from build123d import *

# Parameters (mm, degrees)
BOSS_EXTRU_1_DEPTH      = 22
D_GAGEMENT_M21_D        = 2.4
ESQUISSE5_W             = 22
ESQUISSE5_H             = 10
BOSS_EXTRU_2_DEPTH      = 5
CONG_1_R                = 10
CONG_3_R                = 1
ENL_V_MAT_EXTRU_2_DEPTH = 3
ESQUISSE12_R            = 1.9376057
ENL_V_MAT_EXTRU_3_DEPTH = 37.235341952
ESQUISSE13_R            = 2.5
ENL_V_MAT_EXTRU_4_DEPTH = 2
ESQUISSE15_R            = 2.5
ENL_V_MAT_EXTRU_5_DEPTH = 7


with BuildPart() as part:
    # Esquisse1 → Boss.-Extru.1 (new body)
    with BuildSketch(Plane.XY):
        with BuildLine():
            Line((0, 10), (0, 0))
            Line((0, 0), (6, 0))
            ThreePointArc((6, 0), (11, 5), (16, 0))
            Line((16, 0), (22, 0))
            Line((22, 0), (22, 10))
            Line((22, 10), (0, 10))
        make_face()
    extrude(amount=BOSS_EXTRU_1_DEPTH)

    # Dégagement M21 (through all)
    with Locations(Plane(origin=(0, 10, 0), x_dir=(1, 0, 0), z_dir=(0, 1, 0))):
        with Locations((11, -6), (11, -18), (3, -12), (19, -12)):
            Hole(D_GAGEMENT_M21_D / 2)

    # Esquisse5 → Boss.-Extru.2 (add)
    with BuildSketch(Plane.XY.offset(22)):
        with Locations((11, 5)):
            Rectangle(ESQUISSE5_W, ESQUISSE5_H)
    extrude(amount=BOSS_EXTRU_2_DEPTH)

    # Congé1
    # the kernel refuses this fillet: 10 mm, written as the material it takes off along each edge
    with BuildSketch(Plane(origin=(0, 35, 0), x_dir=(0, 0, 1), z_dir=(0, -1, 0))) as cong_1_piece_1:
        with BuildLine():
            CenterArc((CONG_1_R, -CONG_1_R), CONG_1_R, 90, 90)
            Line((0, -CONG_1_R), (0, 0))
            Line((0, 0), (CONG_1_R, 0))
        make_face()
    extrude(amount=60, mode=Mode.SUBTRACT)
    with BuildSketch(Plane(origin=(0, 35, 27), x_dir=(0, 0, -1), z_dir=(0, -1, 0)), Plane(origin=(22, -25, 0), x_dir=(-1, 0, 0), z_dir=(0, 1, 0)), Plane(origin=(22, -25, 27), x_dir=(0, 0, -1), z_dir=(0, 1, 0))) as cong_1_piece_2:
        with BuildLine():
            CenterArc((CONG_1_R, CONG_1_R), CONG_1_R, 180, 90)
            Line((0, CONG_1_R), (0, 0))
            Line((0, 0), (CONG_1_R, 0))
        make_face()
    extrude(amount=60, mode=Mode.SUBTRACT)

    # Congé3
    cong_3_edges = [part.edges().sort_by_distance(p)[0] for p in [
        (11, 10, 0),
        (0, 10, 13.5),
        (11, 10, 27),
        (22, 10, 13.5),
        (19.071067812, 10, 24.071067812),
        (19.071067812, 10, 2.928932188),
        (2.928932188, 10, 24.071067812),
        (2.928932188, 10, 2.928932188),
    ]]
    fillet(cong_3_edges, radius=CONG_3_R)

    # Esquisse10 → Enlèv. mat.-Extru.2 (cut)
    with BuildSketch(Plane(origin=(0, 0, 22), x_dir=(-1, 0, 0), z_dir=(0, 0, -1))):
        with BuildLine():
            Line((-7, 0), (-15, 0))
            ThreePointArc((-15, 0), (-11, 4), (-7, 0))
        make_face()
    extrude(amount=-ENL_V_MAT_EXTRU_2_DEPTH, mode=Mode.SUBTRACT)

    # Esquisse12 → Enlèv. mat.-Extru.3 (cut, through all)
    with BuildSketch(Plane(origin=(0, 10, 0), x_dir=(1, 0, 0), z_dir=(0, 1, 0))):
        with Locations(Location((11, -23, 0), (0, 0, 270))):
            Circle(ESQUISSE12_R)
    extrude(amount=-ENL_V_MAT_EXTRU_3_DEPTH, mode=Mode.SUBTRACT)

    # Esquisse13 → Enlèv. mat.-Extru.4 (cut)
    with BuildSketch(Plane(origin=(0, 10, 0), x_dir=(1, 0, 0), z_dir=(0, 1, 0))):
        with Locations(Location((11, -12, 0), (0, 0, 270))):
            Circle(ESQUISSE13_R)
    extrude(amount=-ENL_V_MAT_EXTRU_4_DEPTH, mode=Mode.SUBTRACT)

    # Esquisse15 → Enlèv. mat.-Extru.5 (cut)
    with BuildSketch(Plane.XZ):
        with Locations(Location((11, 18, 0), (0, 0, 270))):
            Circle(ESQUISSE15_R)
        with Locations(Location((11, 6, 0), (0, 0, 270))):
            Circle(ESQUISSE15_R)
    extrude(amount=-ENL_V_MAT_EXTRU_5_DEPTH, mode=Mode.SUBTRACT)


solid = part.part
Design review of the part built by this model. Coordinates are the model's own, in mm. A direction names the side the tool comes from. Coordinates: 2 decimals unless noted, no trailing zeros. Order: outer loops, then holes, each group sorted by start corner. A loop starts at its lowest first (then second) coordinate and runs counter-clockwise, first axis right, second up. Notation, with made-up numbers: M 86.5,38.5 L 102.5,38.5 A31 ccw 102.5,77.5 Z; hole C 46.25,60 d5. An arc over 180 degrees is marked long. Use a Markdown table: item, result.
(1) For faces 4 (the cylindrical face through (12.69, 5.94, 19.84)), 5 (the cylindrical face through (19.95, 4.93, 12.73)), 6 (the flat face through (11, 2, 25)), list the 3-axis set-ups (+Z, -Z, +X, -X, +Y, -Y) from which the entire face can be reached by the end or side of a thin tool; tool diameter is ignored.
Worked answers:
| item | result |
|---|---|
| face 4 | -Y |
| face 5 | +Y, -Y |
| face 6 | -Z, -Y |
(2) Add section C-C (x = 11.5). Count the separate pieces of the cut face and the enclosed holes in it, then the cut area to 3 significant figures.
Worked answers:
| item | result |
|---|---|
| separate pieces | 4 |
| enclosed holes | 0 |
| area | 83.8 mm2 |
(3) Wall thickness on probe 1 along Z at (x, y) = (11, 5.1); probe 2 along X at (y, z) = (5.25, 12); probe 3 along X at (y, z) = (3.5, 21.5): over which ranges is each line inside the solid? List them lowest first.
Worked answers:
| item | result |
|---|---|
| probe 1 | z = 0 to 3.5, 8.5 to 15.5, 20.5 to 21.06, 24.94 to 27 |
| probe 2 | x = 0 to 1.8, 4.2 to 17.8, 20.2 to 22 |
| probe 3 | x = 1.07 to 7.43, 14.57 to 20.93 |
(4) Draft analysis for pull direction Z (two halves, no side actions). For faces 1 (the flat face through (4, 0, 14)), 2 (the flat face through (11, 5, 27)), 3 (the cylindrical face through (8.56, 9.01, 11.46)), state which applies: released by +Z, released by -Z, zero draft, split by the parting line, or undercut.
Worked answers:
| item | result |
|---|---|
| face 1 | zero draft |
| face 2 | released by +Z |
| face 3 | undercut |
(5) Add section B-B (y = 6). Give the boundary of the cut face in (x, z).
Worked answers:
| item | result |
|---|---|
| outline | M 0,10 A10 ccw 10,0 L 12,0 A10 ccw 22,10 L 22,17 A10 ccw 12,27 L 10,27 A10 ccw 0,17 Z; hole C 3,12 d2.4; hole C 11,6 d5; hole C 11,18 d5; hole C 11,23 d3.88; hole C 19,12 d2.4 |
(6) For P1, Ø8, axis at x = 11, z = 18, coming from the -Y side; P2, Ø3, axis at x = 3, z = 12, coming from the +Y side; P3, Ø4, axis at x = 11, z = 6, coming from the -Y side; P4, Ø1, axis at x = 15, z = 16.5, coming from the -Y side, all flat-tipped, find the tip position at first contact; note any pin that passes through.
Worked answers:
| item | result |
|---|---|
| P1 | stops at y = 3 |
| P2 | stops at y = 10 |
| P3 | stops at y = 7 |
| P4 | stops at y = 2.18 |
(7) Add section A-A (z = 12). Give the boundary of the cut face in (x, y), then the cut area to 3 significant figures.
Worked answers:
| item | result |
|---|---|
| outline | M 0,0 L 1.8,0 L 1.8,10 L 1,10 A1 ccw 0,9 Z; M 4.2,0 L 6,0 A5 cw 16,0 L 17.8,0 L 17.8,10 L 13.5,10 L 13.5,8 L 8.5,8 L 8.5,10 L 4.2,10 Z; M 20.2,0 L 22,0 L 22,9 A1 ccw 21,10 L 20.2,10 Z |
| area | 122 mm2 |
(8) Add section D-D (y = 0.75). Give the boundary of the cut face in (x, z).
Worked answers:
| item | result |
|---|---|
| outline | M 0,10 A10 ccw 6.06,0.81 L 6.06,22 L 7.07,22 L 7.07,25 L 14.93,25 L 14.93,22 L 15.94,22 L 15.94,0.81 A10 ccw 22,10 L 22,17 A10 ccw 12,27 L 10,27 A10 ccw 0,17 Z; hole C 3,12 d2.4; hole C 19,12 d2.4 |
